Can you work these out from the model? Positions are in its coordinate system, mm. A direction names the side the tool comes from. Round coordinates to 2 decimals unless told otherwise and drop trailing zeros. Loops run counter-clockwise (first coordinate to the right, second up) from the corner with the lowest first, then second, coordinate; pieces in that order, holes last.
Solid Edge part; units mm, degrees
sketch "Sketch1" plane through (0, 0, 0) normal (0, 0, 1) x (1, 0, 0)
  circle A0 centre (0, 0) radius 9.28
extrude "Protrusion1" add sketch "Sketch1" along normal blind 6.63
sketch "Sketch2" plane through (0, 0, 0) normal (0, 0, -1) x (1, 0, 0)
  circle A0 centre (0, 0) radius 5
extrude "Protrusion2" add sketch "Sketch2" along normal blind 30
sketch "Sketch3" plane through (0, 0, -30) normal (0, 0, -1) x (1, 0, 0)
  circle A0 centre (0, 0) radius 4.9997
extrude "Cutout1" cut sketch "Sketch3" against normal blind 26 flip side to cut
chamfer "Chamfer_1" distance 0.75 angle 45 1 edges at (-4.9997, 0, -30)
sketch "Sketch4" plane through (0, 0, 6.63) normal (0, 0, 1) x (1, 0, 0)
  line L0 (-4.703, 8) -> (4.703, 8)
extrude "Cutout2" cut sketch "Sketch4" against normal up to next material side at (0, 8.05, 6.63)
pattern_circular "Pattern1" count 6 over 360 about axis through (0, 0, 6.63) along (0, 0, 1) of "Cutout2"
properties part number "24101206"
(1) If we section it at C-C, the plane y = 6.75: List the corners of the cut face in (x, z) for me, then the cut area to 3 significant figures.
Worked answers:
outline: (-5.34, 0) - (5.34, 0) - (5.34, 6.63) - (-5.34, 6.63) - close
area: 70.8 mm2
(2) For faces 1 (the cylindrical face through (-1.08, -4.88, -1.97)), 2 (the flat face through (0, 0, -30)), which set-ups out of +Z, -Z, +X, -X, +Y, -Y let a thin tool reach every point of the face, with its end or its side?
Worked answers:
face 1: -Z
face 2: -Z, +X, -X, +Y, -Y
(3) If we section it at B-B, the plane z = -0.5: List the corners of the cut face in (x, y) for me.
Worked answers:
outline: circle Ø10 at (0, 0)
(4) If I drill on line 1 (Z direction, x = -4.5, y = -5.25); line 2 (X direction, y = -1, z = -15.5); line 3 (X direction, y = -2.5, z = 5.5), over which ranges is the centre line in solid material (lowest first)?
Worked answers:
line 1: z = 0 to 6.63
line 2: x = -4.9 to 4.9
line 3: x = -7.79 to 7.79
